Source: CAD feature listing. Evaluate the final solid. Frame: model axes, mm. A direction names the side the tool comes from. Give positions to 0.01 mm unless a question says otherwise; leave off trailing zeros. Write each loop counter-clockwise with the first axis right and the second up, starting at its lowest first coordinate (ties: lowest second). Pieces come first, ordered by that corner, then holes. Notation, with made-up numbers: (51, -11) -> (110, -11) arc R25 ccw to (110, 17) -> close; hole circle Ø4 at (-2, 5). An arc over 180 degrees is marked (long way). Use one line per item in the form item = value. Start each with the question number.
(1) Set-up query: faces 1 (the face through (-2.89, -181.52, -0.33)), 2 (the face through (2, -95, 0)). Return all of +Z, -Z, +X, -X, +Y, -Y with unobstructed straight access to the full face (end or side cutting, diameter ignored); none if empty.
(2) Cut plane B-B, the plane y = -49.5. Output: boundary loops of the cut face in (x, z), and give its area (3 significant figures).
(3) Cut plane A-A, the plane y = -72. Output: boundary loops of the cut face in (x, z), and give its area (3 significant figures).
(4) Draft query along Z for faces 3 (the face through (2.86, -133.52, -0.33)), 4 (the face through (0, -95, -4)), 5 (the face through (2.86, -42.44, -0.54)), 6 (the face through (-3.75, -95, 0)). Return one class per face: pulls with the +Z half, pulls with the -Z half, needs draft (parallel to the pull), parting line crosses it, or undercut.
(5) First-contact query: P1, Ø3, axis at y = -40, z = 0, coming from the -X side. Flat tip, straight axial feed; report the tip coordinate or a pass-through.
(6) Material intervals for line 1 along X through (y, z) = (-141, 2); line 2 along Z through (x, y) = (3.4, -184); line 3 along Z through (x, y) = (-0.5, -21), sorted ascending. Write a range as from..to.
(7) Cut plane C-C, the plane z = 0. Count the separate pieces of the cut face and the enclosed holes in it, and give its area (3 significant figures).
from build123d import *

# Parameters (mm, degrees)
BASE_DEPTH  = 192
ESQUISSE2_R = 2.5
TROU_DEPTH  = 193.188058942


with BuildPart() as part:
    # Esquisse1 → Base (new body)
    with BuildSketch(Plane(origin=(0, 0, 0), x_dir=(1, 0, 0), z_dir=(0, 1, 0))):
        Polygon((-2, -4), (-2, 3), (2, 3), (2, -4), (3.75, -4), (3.75, 4), (-3.75, 4), (-3.75, -4), align=None)
    extrude(amount=-BASE_DEPTH)

    # Esquisse2 → Trou (cut, through all)
    with BuildSketch(Plane.ZY.offset(3.75)):
        with Locations((0, -8)):
            Circle(ESQUISSE2_R)
        with Locations((0, -24)):
            Circle(ESQUISSE2_R)
        with Locations((0, -40)):
            Circle(ESQUISSE2_R)
        with Locations((0, -56)):
            Circle(ESQUISSE2_R)
        with Locations((0, -72)):
            Circle(ESQUISSE2_R)
        with Locations((0, -88)):
            Circle(ESQUISSE2_R)
        with Locations((0, -104)):
            Circle(ESQUISSE2_R)
        with Locations((0, -120)):
            Circle(ESQUISSE2_R)
        with Locations((0, -136)):
            Circle(ESQUISSE2_R)
        with Locations((0, -152)):
            Circle(ESQUISSE2_R)
        with Locations((0, -168)):
            Circle(ESQUISSE2_R)
        with Locations((0, -184)):
            Circle(ESQUISSE2_R)
    extrude(amount=-TROU_DEPTH, mode=Mode.SUBTRACT)


solid = part.part
Geometry says:
q1.face_1 = +X, -X
q1.face_2 = +Z, +Y, -Y
q2.outline = (-3.75, -4) -> (3.75, -4) -> (3.75, 4) -> (2, 4) -> (2, -3) -> (-2, -3) -> (-2, 4) -> (-3.75, 4) -> close
q2.area = 32.0 mm^2
q3.outline = (-3.75, -4) -> (3.75, -4) -> (3.75, -2.5) -> (2, -2.5) -> (2, -3) -> (-2, -3) -> (-2, -2.5) -> (-3.75, -2.5) -> close; (-3.75, 2.5) -> (-2, 2.5) -> (-2, 4) -> (-3.75, 4) -> close; (2, 2.5) -> (3.75, 2.5) -> (3.75, 4) -> (2, 4) -> close
q3.area = 14.5 mm^2
q4.face_3 = undercut
q4.face_4 = pulls with the -Z half
q4.face_5 = undercut
q4.face_6 = needs draft
q5.P1 = through
q6.line_1 = -3.75..-2, 2..3.75
q6.line_2 = -4..-2.5, 2.5..4
q6.line_3 = -4..-3
q7.separate_pieces = 26
q7.enclosed_holes = 0
q7.area = 462 mm^2
